from build123d import *

# Parameters (mm, degrees)
SKETCH1_W            = 22.5
SKETCH1_H            = 25
SKETCH1_R            = 7.5
BOSS_EXTRUDE1_DEPTH  = 24
CUT_EXTRUDE4_DEPTH   = 30.807717122
SKETCH7_W            = 10
SKETCH7_H            = 25
BOSS_EXTRUDE2_DEPTH  = 24
SKETCH8_R            = 4.1
CUT_EXTRUDE5_DEPTH   = 48
SKETCH135_W          = 19.5
SKETCH135_H          = 24
BOSS_EXTRUDE66_DEPTH = 15
BOSS_EXTRUDE67_DEPTH = 10
SKETCH137_W          = 6.5
SKETCH137_H          = 24
CUT_EXTRUDE6_DEPTH   = 5.3
SKETCH138_W          = 6.5
SKETCH138_H          = 1.8
BOSS_EXTRUDE68_DEPTH = 24
SKETCH139_W          = 6.5
SKETCH139_H          = 13.5
SKETCH139_R          = 1.6
BOSS_EXTRUDE69_DEPTH = 5


with BuildPart() as part:
    # Sketch1 → Boss-Extrude1 (new body)
    with BuildSketch(Plane(origin=(0, 0, 0), x_dir=(1, 0, 0), z_dir=(0, 1, 0))):
        with Locations((1.25, 0)):
            Rectangle(SKETCH1_W, SKETCH1_H)
        with Locations(Location((0, 0, 0), (0, 0, 270))):
            Circle(SKETCH1_R, mode=Mode.SUBTRACT)
    extrude(amount=BOSS_EXTRUDE1_DEPTH)

    # Sketch5 → Cut-Extrude4 (cut, through all)
    with BuildSketch(Plane.XZ):
        Polygon((12.5, 12.5), (6.5, 12.5), (6.5, 4.363484846), (6.1, 4.363484846), (6.1, -4.363484846), (6.5, -4.363484846), (6.5, -12.5), (12.5, -12.5), align=None)
    extrude(amount=-CUT_EXTRUDE4_DEPTH, mode=Mode.SUBTRACT)

    # Sketch7 → Boss-Extrude2 (add)
    with BuildSketch(Plane.XZ):
        with Locations((-15, 0)):
            Rectangle(SKETCH7_W, SKETCH7_H)
    extrude(amount=-BOSS_EXTRUDE2_DEPTH)

    # Sketch8 → Cut-Extrude5 (cut)
    with BuildSketch(Plane.XY.offset(12.5)):
        with Locations((-14, 12)):
            Circle(SKETCH8_R)
    extrude(amount=-CUT_EXTRUDE5_DEPTH, mode=Mode.SUBTRACT)

    # Sketch135 → Boss-Extrude66 (add)
    with BuildSketch(Plane(origin=(0, 0, -12.5), x_dir=(-1, 0, 0), z_dir=(0, 0, -1))):
        with Locations((29.75, 12)):
            Rectangle(SKETCH135_W, SKETCH135_H)
    extrude(amount=-BOSS_EXTRUDE66_DEPTH)

    # Sketch136 → Boss-Extrude67 (add)
    with BuildSketch(Plane.XY.offset(2.5)):
        with BuildLine():
            Line((-26.5, 0), (-30.65, 0))
            Line((-30.65, 0), (-32.618157491, 0))
            Line((-32.618157491, 0), (-31.015837104, 1.142896884))
            ThreePointArc((-31.015837104, 1.142896884), (-29.165912572, 3.280355677), (-28.5, 6.027629109))
            Line((-28.5, 6.027629109), (-28.5, 24))
            Line((-28.5, 24), (-26.5, 24))
            Line((-26.5, 24), (-26.5, 0))
        make_face()
        with BuildLine():
            Line((-31, 24), (-39.5, 24))
            Line((-39.5, 24), (-39.5, 8.68))
            Line((-39.5, 8.68), (-39.5, 6.362551494))
            Line((-39.5, 6.362551494), (-38.492686138, 8.449627525))
            ThreePointArc((-38.492686138, 8.449627525), (-37.750547948, 9.507229314), (-36.71, 10.273095232))
            Line((-36.71, 10.273095232), (-31, 13.19))
            Line((-31, 13.19), (-31, 24))
        make_face()
        with BuildLine():
            Line((-30.2, 5.530404879), (-30.2, 11.689701848))
            Line((-30.2, 11.689701848), (-35.685050881, 8.887710417))
            ThreePointArc((-35.685050881, 8.887710417), (-35.938141024, 2.314923436), (-30.2, 5.530404879))
        make_face()
    extrude(amount=BOSS_EXTRUDE67_DEPTH)

    # Sketch137 → Cut-Extrude6 (cut)
    with BuildSketch(Plane.XY.offset(2.5)):
        with Locations((-23.25, 12)):
            Rectangle(SKETCH137_W, SKETCH137_H)
    extrude(amount=-CUT_EXTRUDE6_DEPTH, mode=Mode.SUBTRACT)

    # Sketch138 → Boss-Extrude68 (add)
    with BuildSketch(Plane.XZ):
        with Locations((-23.25, 11.6)):
            Rectangle(SKETCH138_W, SKETCH138_H)
    extrude(amount=-BOSS_EXTRUDE68_DEPTH)

    # Sketch139 → Boss-Extrude69 (add)
    with BuildSketch(Plane(origin=(0, 24, 0), x_dir=(1, 0, 0), z_dir=(0, 1, 0))):
        with Locations((-23.25, -3.95)):
            Rectangle(SKETCH139_W, SKETCH139_H)
        with Locations(Location((-23.25, -3.95, 0), (0, 0, 270))):
            Circle(SKETCH139_R, mode=Mode.SUBTRACT)
    extrude(amount=-BOSS_EXTRUDE69_DEPTH)


solid = part.part
Input: part model. Units: mm. Frame: model coordinates. A direction names the side the tool comes from. Round coordinates to 2 decimals unless told otherwise and drop trailing zeros. Order: outer loops, then holes, each group sorted by start corner. A loop starts at its lowest first (then second) coordinate and runs counter-clockwise, first axis right, second up. Notation, with made-up numbers: (-10.5, -10) - (21.5, -10) arc R24 cw to (21.5, 8) - close; hole circle Ø10 at (-23, 37). An arc over 180 degrees is marked (long way). Answer as a JSON object with one key per item and string values. Group by question number.
(1) Draft query along Z for faces 5 (the face through (-26.5, 10, 4)), 6 (the face through (-20, 9, 4)), 7 (the face through (-31, 19, 7)), 8 (the face through (-21, 12, -12.5)). Return one class per face: released by +Z, released by -Z, zero draft, split by the parting line, or undercut.
(2) Cut plane A-A (z = 8.25). Return loops of the section in (x, y), then the cut area to 3 significant figures.
(3) Material intervals for probe 1 along X at (y, z) = (16.25, 9); probe 2 along Z at (x, y) = (-21, 7); probe 3 along X at (y, z) = (22.25, 8.5), sorted ascending. Write a range as from..to.
(4) Pin query (flat end, axial travel): P1, Ø2.5, axis at x = -23.25, z = 3.95, coming from the +Y side; P2, Ø2, axis at x = -22.5, z = 2, coming from the -Y side. Return the tip coordinate at first contact, or that it passes through.
(5) Cut plane C-C (y = 19.5). Return loops of the section in (x, z), then the cut area to 3 significant figures.
(6) Cut plane B-B (x = -23.25). Return loops of the section in (y, z).
(7) Cut plane D-D (y = 9.5). Return loops of the section in (x, z), then the cut area to 3 significant figures.
(8) Reachability of faces 1 (the face through (-39, 7.4, 7.4)), 2 (the face through (-23, 9, 10.7)), 3 (the face through (-28.5, 15, 7)), 4 (the face through (-32.9, 10.31, 7.43)) from +Z, -Z, +X, -X, +Y, -Y: full face, straight path, thin tool, end or side. Return the list, or none.
Here are the results:
{
 "1": {"face 5": "undercut", "face 6": "undercut", "face 7": "zero draft", "face 8": "released by -Z"},
 "2": {"outline": "(-39.5, 6.36) - (-38.49, 8.45) arc R4 cw to (-36.71, 10.27) - (-31, 13.19) - (-31, 24) - (-39.5, 24) - close; (-35.69, 8.89) arc R3.77 ccw (long way) to (-30.2, 5.53) - (-30.2, 11.69) - close; (-32.62, 0) - (-26.5, 0) - (-26.5, 19) - (-20, 19) - (-20, 0) - (6.5, 0) - (6.5, 24) - (-28.5, 24) - (-28.5, 6.03) arc R6 cw to (-31.02, 1.14) - close; hole circle Ø8.2 at (-14, 12)", "area": "837 mm^2"},
 "3": {"probe 1": "x = -39.5..-31, -28.5..-26.5, -20..6.5", "probe 2": "z = -12.5..-2.8, 10.7..12.5", "probe 3": "x = -39.5..-31, -28.5..6.5"},
 "4": {"P1": "passes through", "P2": "stops at y = 19"},
 "5": {"outline": "(-39.5, -12.5) - (6.5, -12.5) - (6.5, -4.36) - (6.1, -4.36) arc R7.5 cw (long way) to (6.1, 4.36) - (6.5, 4.36) - (6.5, 12.5) - (-28.5, 12.5) - (-28.5, 2.5) - (-31, 2.5) - (-31, 12.5) - (-39.5, 12.5) - close; hole circle Ø3.2 at (-23.25, 3.95)", "area": "945 mm^2"},
 "6": {"outline": "(0, -12.5) - (24, -12.5) - (24, 2.35) - (19, 2.35) - (19, -2.8) - (0, -2.8) - close; (0, 10.7) - (19, 10.7) - (19, 5.55) - (24, 5.55) - (24, 12.5) - (0, 12.5) - close"},
 "7": {"outline": "(-39.5, -12.5) - (-17.25, -12.5) - (-17.25, 12.5) - (-28.5, 12.5) - (-28.5, 2.5) - (-30.2, 2.5) - (-30.2, 12.5) - (-34.49, 12.5) - (-34.49, 2.5) - (-37.76, 2.5) - (-37.76, 12.5) - (-39.5, 12.5) - close; (-10.75, -12.5) - (6.5, -12.5) - (6.5, -4.36) - (6.1, -4.36) arc R7.5 cw (long way) to (6.1, 4.36) - (6.5, 4.36) - (6.5, 12.5) - (-10.75, 12.5) - close; hole (-26.5, -2.8) - (-20, -2.8) - (-20, 10.7) - (-26.5, 10.7) - close", "area": "678 mm^2"},
 "8": {"face 1": "+Z, -Y", "face 2": "-Y", "face 3": "+Z, +Y", "face 4": "+Z"}
}
